from build123d import *

# Parameters (mm, degrees)
F0_W     = 280
F0_H     = 600
F1_DEPTH = 2
F2_W     = 3
F2_H     = 600
F3_DEPTH = 9
F4_W     = 50
F4_H     = 57.932376
F5_DEPTH = 4
F7_DEPTH = 250
F8_W     = 35
F8_H     = 57.431721
F9_DEPTH = 4


with BuildPart() as f1:
    # F0 (on Top) → F1 (new body, symmetric)
    with BuildSketch(Plane.XY):
        Rectangle(F0_W, F0_H)
    extrude(amount=F1_DEPTH, both=True)

    # F2 (on face) → F3 (join)
    with BuildSketch(Plane.XY.offset(2)):
        with Locations((-138.5, 0)):
            Rectangle(F2_W, F2_H)
        with Locations((138.5, 0)):
            Rectangle(F2_W, F2_H)
    extrude(amount=F3_DEPTH)

    # F4 (on Top) → F5 (join)
    with BuildSketch(Plane.XY):
        with Locations((-164.812601, 250.6136)):
            Rectangle(F4_W, F4_H)
        with Locations((164.812601, 250.6136)):
            Rectangle(F4_W, F4_H)
        with Locations((-164.812601, -250.6136)):
            Rectangle(F4_W, F4_H)
        with Locations((164.812601, -250.6136)):
            Rectangle(F4_W, F4_H)
    extrude(amount=F5_DEPTH)

    # F6 (on Top) → F7 (join)
    with BuildSketch(Plane.XY):
        Polygon((-189.361796, 222.509515), (-189.361796, 279.471008), (-194.60392, 279.439882), (-194.60392, 222.509515), align=None)
        Polygon((194.60392, 222.509515), (194.60392, 279.439882), (189.361796, 279.471008), (189.361796, 222.509515), align=None)
        Polygon((194.60392, -222.509515), (189.361796, -222.509515), (189.361796, -279.471008), (194.60392, -279.439882), align=None)
        Polygon((-194.60392, -222.509515), (-194.60392, -279.439882), (-189.361796, -279.471008), (-189.361796, -222.509515), align=None)
    extrude(amount=F7_DEPTH)

    # F8 (on face) → F9 (join)
    with BuildSketch(Plane.XY.offset(250)):
        with Locations((-206.861796, 250.755147)):
            Rectangle(F8_W, F8_H)
        with Locations((206.861796, 250.755147)):
            Rectangle(F8_W, F8_H)
        with Locations((206.861796, -250.755147)):
            Rectangle(F8_W, F8_H)
        with Locations((-206.861796, -250.755147)):
            Rectangle(F8_W, F8_H)
    extrude(amount=F9_DEPTH)


solid = f1.part
Geometry: final body of the model. Coordinates: model frame, mm. A direction names the side the tool comes from. Give positions to 0.01 mm unless a question says otherwise; leave off trailing zeros. Write each loop counter-clockwise with the first axis right and the second up, starting at its lowest first coordinate (ties: lowest second). Pieces come first, ordered by that corner, then holes. Notation, with made-up numbers: (42.5, -25) - (84.5, -25) arc R26 cw to (84.5, 6) - close; hole circle Ø7 at (-25, 4.5). An arc over 180 degrees is marked (long way). Return JSON: item names as keys, results as strings. Group by question number.
1) Section B-B on y = 101.5. Return the cut outline in (x, z).
2) Section C-C on x = 14.5. Return the cut outline in (y, z), plus the area to 3 significant figures.
3) Set-up query: faces 1 (the flat face through (189.362, 251, 127)), 2 (the flat face through (167, 251, 0)), 3 (the flat face through (-1, 300, 0)). Return all of +Z, -Z, +X, -X, +Y, -Y with unobstructed straight access to the full face (end or side cutting, diameter ignored); none if empty.
4) Mould query, pull axis X, two halves, no side actions, for faces 4 (the flat face through (-194.604, -251, 123)), 5 (the flat face through (-189.362, -251, 127)), 6 (the flat face through (207, -250, 254)). Classes: released by +X, released by -X, zero draft, split by the parting line, or undercut.
5) First-contact query: P1, Ø1.2, axis at x = 201, z = 251.5, coming from the +Y side; P2, Ø3, axis at x = -210, z = 252, coming from the -Y side; P3, Ø0.7, axis at y = 222, z = 1, coming from the -X side. Flat tips, straight axial feed; report the tip coordinate or a pass-through.
6) Section A-A on z = 198.5. Return the cut outline in (x, y), plus the area to 3 significant figures.
7) Line query: line 1 (X direction, y = -246.5, z = 228.5); line 2 (Z direction, x = 13, y = 231); line 3 (Y direction, x = -190, z = 28). Output: solid intervals per line, ascending.
8) Section D-D on y = 251.5. Return the cut outline in (x, z).
Filled in:
{
 "1": {"outline": "(-140, -2) - (140, -2) - (140, 11) - (137, 11) - (137, 2) - (-137, 2) - (-137, 11) - (-140, 11) - close"},
 "2": {"outline": "(-300, -2) - (300, -2) - (300, 2) - (-300, 2) - close", "area": "2,400 mm^2"},
 "3": {"face 1": "+Z, +Y, -Y", "face 2": "-Z, +X, +Y, -Y", "face 3": "+Z, -Z, +X, -X, +Y"},
 "4": {"face 4": "released by -X", "face 5": "undercut", "face 6": "zero draft"},
 "5": {"P1": "stops at y = 279.47", "P2": "stops at y = -279.47", "P3": "stops at x = -189.81"},
 "6": {"outline": "(-194.6, -279.44) - (-189.36, -279.47) - (-189.36, -222.51) - (-194.6, -222.51) - close; (-194.6, 222.51) - (-189.36, 222.51) - (-189.36, 279.47) - (-194.6, 279.44) - close; (189.36, -279.47) - (194.6, -279.44) - (194.6, -222.51) - (189.36, -222.51) - close; (189.36, 222.51) - (194.6, 222.51) - (194.6, 279.44) - (189.36, 279.47) - close", "area": "1,190 mm^2"},
 "7": {"line 1": "x = -194.6 to -189.36, 189.36 to 194.6", "line 2": "z = -2 to 2", "line 3": "y = -279.47 to -222.51, 222.51 to 279.47"},
 "8": {"outline": "(-224.36, 250) - (-194.6, 250) - (-194.6, 0) - (-140, 0) - (-140, -2) - (140, -2) - (140, 0) - (194.6, 0) - (194.6, 250) - (224.36, 250) - (224.36, 254) - (189.36, 254) - (189.36, 4) - (140, 4) - (140, 11) - (137, 11) - (137, 2) - (-137, 2) - (-137, 11) - (-140, 11) - (-140, 4) - (-189.36, 4) - (-189.36, 254) - (-224.36, 254) - close"}
}
